Model file for the job. Use its own axes, mm. A direction names the side the tool comes from. Round coordinates to 2 decimals unless told otherwise and drop trailing zeros. Loops run counter-clockwise (first coordinate to the right, second up) from the corner with the lowest first, then second, coordinate; pieces in that order, holes last. Notation, with made-up numbers: M 9,-27 L 14,-27 A10 ccw 14,-23 Z; hole C 1,-7 d9. An arc over 180 degrees is marked long. Use a Markdown table: item, result. Add a question column.
Q1. Probe line 1 (X direction, y = 2.25, z = 14.5); line 2 (Y direction, x = -18.25, z = 8); line 3 (X direction, y = -0.25, z = 22.5). List the from-to ranges inside material, lowest first. Write a range as from..to.
Q2. Pin check, flat tips, straight feed: pin 1 (3 mm diameter, centred on y = 17.52, z = 38.24, fed in from -X); pin 2 (1.5 mm diameter, centred on x = -5.5, z = 27.5, fed in from +Y); pin 3 (5 mm diameter, centred on y = 19, z = 20, fed in from -X). Stop position of each tip, or through.
Q3. Tool access for faces 1 (the face through (-12, 0, 21)), 2 (the face through (-20.9, -0.9, 41.6)): list every direction of +Z, -Z, +X, -X, +Y, -Y with a clear straight run to the whole face (end or side of a thin tool).
Q4. Mould opens along Z. For faces 3 (the face through (0.8, 20.9, 41.6)), 4 (the face through (-22.286, -1, 21)), 5 (the face through (-18.507, -0.843, 6.305)), 6 (the face through (-20.854, -0.867, 1.358)) say: +Z half, -Z half, draft (parallel to the pull), parting line (faces both ways), or undercut.
Q5. Cut at C-C (y = 14). Give the cut face in (x, z).
Q6. Cut at A-A (z = 3.5). Give the cut face in (x, y), plus the area to 3 significant figures.
Q7. Cut at D-D (x = -13). Give the cut face in (y, z).
Q8. Cut at B-B (z = 31.5). Give the cut face in (x, y), plus the area to 3 significant figures.
from build123d import *

# Parameters (mm, degrees)
F1_DEPTH = 43.005985
F2_R     = 1.98374
F3_R     = 3.69316
F4_R     = 1.8288
F5_DEPTH = 1.70942
F6_R     = 1.8288
F7_DEPTH = 1.70942
F8_R     = 4.7625


with BuildPart() as f1:
    # F0 (on Top) → F1 (new body)
    with BuildSketch(Plane.XY):
        Polygon((1.70942, 22.28596), (0, 22.28596), (0, 0), (-22.28596, 0), (-22.28596, -1.70942), (1.70942, -1.70942), align=None)
    extrude(amount=F1_DEPTH)

    # F2
    f2_edges = [f1.edges().sort_by_distance(p)[0] for p in [
        (0, 0, 21.502992),
    ]]
    fillet(f2_edges, radius=F2_R)

    # F3
    f3_edges = [f1.edges().sort_by_distance(p)[0] for p in [
        (1.70942, -1.70942, 21.502992),
    ]]
    fillet(f3_edges, radius=F3_R)

    # F4 (on face) → F5 (cut, through all)
    with BuildSketch(Plane(origin=(0, 0, 0), x_dir=(0, -1, 0), z_dir=(-1, 0, 0))):
        with Locations((-17.52346, 38.243485)):
            Circle(F4_R)
        with Locations((-17.52346, 4.7625)):
            Circle(F4_R)
    extrude(amount=-F5_DEPTH, mode=Mode.SUBTRACT)

    # F6 (on face) → F7 (cut, through all)
    with BuildSketch(Plane(origin=(0, 0, 0), x_dir=(-1, 0, 0), z_dir=(0, 1, 0))):
        with Locations((17.52346, 38.243485)):
            Circle(F6_R)
        with Locations((17.52346, 4.7625)):
            Circle(F6_R)
    extrude(amount=-F7_DEPTH, mode=Mode.SUBTRACT)

    # F8
    f8_edges = [f1.edges().sort_by_distance(p)[0] for p in [
        (0.85471, 22.28596, 43.005985),
        (-22.28596, -0.85471, 43.005985),
        (-22.28596, -0.85471, 0),
        (0.85471, 22.28596, 0),
    ]]
    fillet(f8_edges, radius=F8_R)


solid = f1.part
Checked values:
| question | item | result |
|---|---|---|
| 1 | line 1 | x = 0..1.71 |
| 1 | line 2 | y = -1.71..0 |
| 1 | line 3 | x = -22.29..0.96 |
| 2 | pin 1 | passes through |
| 2 | pin 2 | stops at y = 0 |
| 2 | pin 3 | stops at x = 0 |
| 3 | face 1 | +Z, -Z, -X, +Y |
| 3 | face 2 | +Z, -X, +Y, -Y |
| 4 | face 3 | +Z half |
| 4 | face 4 | draft |
| 4 | face 5 | undercut |
| 4 | face 6 | -Z half |
| 5 | outline | M 0,0 L 1.71,0 L 1.71,43.01 L 0,43.01 Z |
| 6 | outline | M -22.12,-1.71 L -18.85,-1.71 L -18.85,0 L -22.12,0 Z; M -16.2,-1.71 L -1.98,-1.71 A3.69 ccw 1.71,1.98 L 1.71,16.2 L 0,16.2 L 0,1.98 A1.98 cw -1.98,0 L -16.2,0 Z; M 0,18.85 L 1.71,18.85 L 1.71,22.12 L 0,22.12 Z |
| 6 | area | 67.4 mm^2 |
| 7 | outline | M -1.71,0 L 0,0 L 0,43.01 L -1.71,43.01 Z |
| 8 | outline | M -22.29,-1.71 L -1.98,-1.71 A3.69 ccw 1.71,1.98 L 1.71,22.29 L 0,22.29 L 0,1.98 A1.98 cw -1.98,0 L -22.29,0 Z |
| 8 | area | 77.0 mm^2 |
